from build123d import *

# Parameters (mm, degrees)
BOSS_EXTRUDE1_DEPTH = 26
FILLET1_R           = 2
SKETCH2_R           = 1.6
CUT_EXTRUDE1_DEPTH  = 13.5
SKETCH3_R           = 1.6
CUT_EXTRUDE2_DEPTH  = 13.5


with BuildPart() as part:
    # Sketch1 → Boss-Extrude1 (new body, symmetric)
    with BuildSketch(Plane.XY):
        Polygon((62, 0), (62, 2.5), (-12.5, 2.5), (-12.5, 0), (-8.95, 0), (-8.95, -1), (-6.05, -1), (-6.05, 0), (-2.5, 0), (-2.5, -3.55), (-3.5, -3.55), (-3.5, -6.45), (-2.5, -6.45), (-2.5, -10), (0, -10), (0, 0), align=None)
    extrude(amount=BOSS_EXTRUDE1_DEPTH, both=True)

    # Fillet1
    fillet1_edges = [part.edges().sort_by_distance(p)[0] for p in [
        (0, 0, 0),
    ]]
    fillet(fillet1_edges, radius=FILLET1_R)

    # Sketch2 → Cut-Extrude1 (cut, through all)
    with BuildSketch(Plane(origin=(0, 0, 0), x_dir=(0, 0, -1), z_dir=(1, 0, 0))):
        with Locations((0, -5)):
            Circle(SKETCH2_R)
    extrude(amount=-CUT_EXTRUDE1_DEPTH, mode=Mode.SUBTRACT)

    # Sketch3 → Cut-Extrude2 (cut, through all)
    with BuildSketch(Plane(origin=(0, 2.5, 0), x_dir=(1, 0, 0), z_dir=(0, 1, 0))):
        with Locations((-7.5, 0)):
            Circle(SKETCH3_R)
    extrude(amount=-CUT_EXTRUDE2_DEPTH, mode=Mode.SUBTRACT)


solid = part.part
Verification items for the finished model (mm, model axes). A direction names the side the tool comes from. Give positions to 0.01 mm unless a question says otherwise; leave off trailing zeros. Write each loop counter-clockwise with the first axis right and the second up, starting at its lowest first coordinate (ties: lowest second). Pieces come first, ordered by that corner, then holes. Notation, with made-up numbers: M 16,-18.75 L 33,-18.75 A24 ccw 33,-6.75 Z; hole C -22.5,-7 d3. An arc over 180 degrees is marked long. Put each result on its own line as item: value. Start each with the question number.
1. Section check D-D (x = 23.5). Record the cut outline in (y, z), and give its area (3 significant figures).
2. Scan lines: line 1 along Z through (x, y) = (-7.5, 1.4); line 2 along Y through (x, z) = (-0.8, 0); line 3 along X through (y, z) = (1.8, 0). Record each from-to range of solid material in increasing order. Write a range as [from, to].
3. Set-up check for faces 1 (the face through (0, -7, 0)), 2 (the face through (-3.5, -5, 14)), 3 (the face through (19, 1, 26)): record each of +Z, -Z, +X, -X, +Y, -Y from which the full face is reachable in a straight line by a thin tool's end or side.
4. Section check C-C (z = -3). Record the cut outline in (x, y), and give its area (3 significant figures).
5. Section check B-B (x = -7.5). Record the cut outline in (y, z).
6. Draft check along X on faces 4 (the face through (-8, -1, 14)), 5 (the face through (-2.5, -2, 0)), 6 (the face through (-3.5, -5, -13)). Enter one of: +X half, -X half, draft (parallel to the pull), parting line (faces both ways), or undercut.
7. Go/stop test with flat-tipped pins: pin 1 Ø0.5 at (y, z) = (-0.5, 12) entering from -X; pin 2 Ø1.8 at (x, z) = (-10.5, -3) entering from -Y; pin 3 Ø2 at (y, z) = (-4.5, 18) entering from -X. Record where each tip stops, or that it passes through.
8. Section check A-A (y = -5). Record the cut outline in (x, z).
Answer list:
1. outline: M 0,-26 L 2.5,-26 L 2.5,26 L 0,26 Z
1. area: 130 mm2
2. line 1: [-26, -1.6], [1.6, 26]
2. line 2: [-10, -6.6], [-3.4, 2.5]
2. line 3: [-12.5, -9.1], [-5.9, 62]
3. face 1: +Z, -Z, +X, -Y
3. face 2: +Z, -Z, -X, -Y
3. face 3: +Z, +X, -X, +Y, -Y
4. outline: M -12.5,0 L -8.95,0 L -8.95,-1 L -6.05,-1 L -6.05,0 L -2.5,0 L -2.5,-3.55 L -3.5,-3.55 L -3.5,-6.45 L -2.5,-6.45 L -2.5,-10 L 0,-10 L 0,-2 A2 cw 2,0 L 62,0 L 62,2.5 L -12.5,2.5 Z
4. area: 218 mm2
5. outline: M -1,-26 L 2.5,-26 L 2.5,-1.6 L -1,-1.6 Z; M -1,1.6 L 2.5,1.6 L 2.5,26 L -1,26 Z
6. face 4: draft
6. face 5: undercut
6. face 6: -X half
7. pin 1: x = -8.95
7. pin 2: y = 0
7. pin 3: x = -3.5
8. outline: M -3.5,-26 L 0,-26 L 0,-1.6 L -3.5,-1.6 Z; M -3.5,1.6 L 0,1.6 L 0,26 L -3.5,26 Z
